Could you check a few things on this drawing? It's one solid part, dimensions in mm from its lowest x, y, z. Give positions to 0.01 mm unless a question says otherwise; leave off trailing zeros. Loops run counter-clockwise (first coordinate to the right, second up) from the corner with the lowest first, then second, coordinate; pieces in that order, holes last. Notation, with made-up numbers: M 50,81.5 L 96,81.5 A21 ccw 96,111.5 Z; hole C 44.25,-7.5 d9. An arc over 180 degrees is marked long. Write each question's results on one line, items separated by ' | '. Start each with the question number.
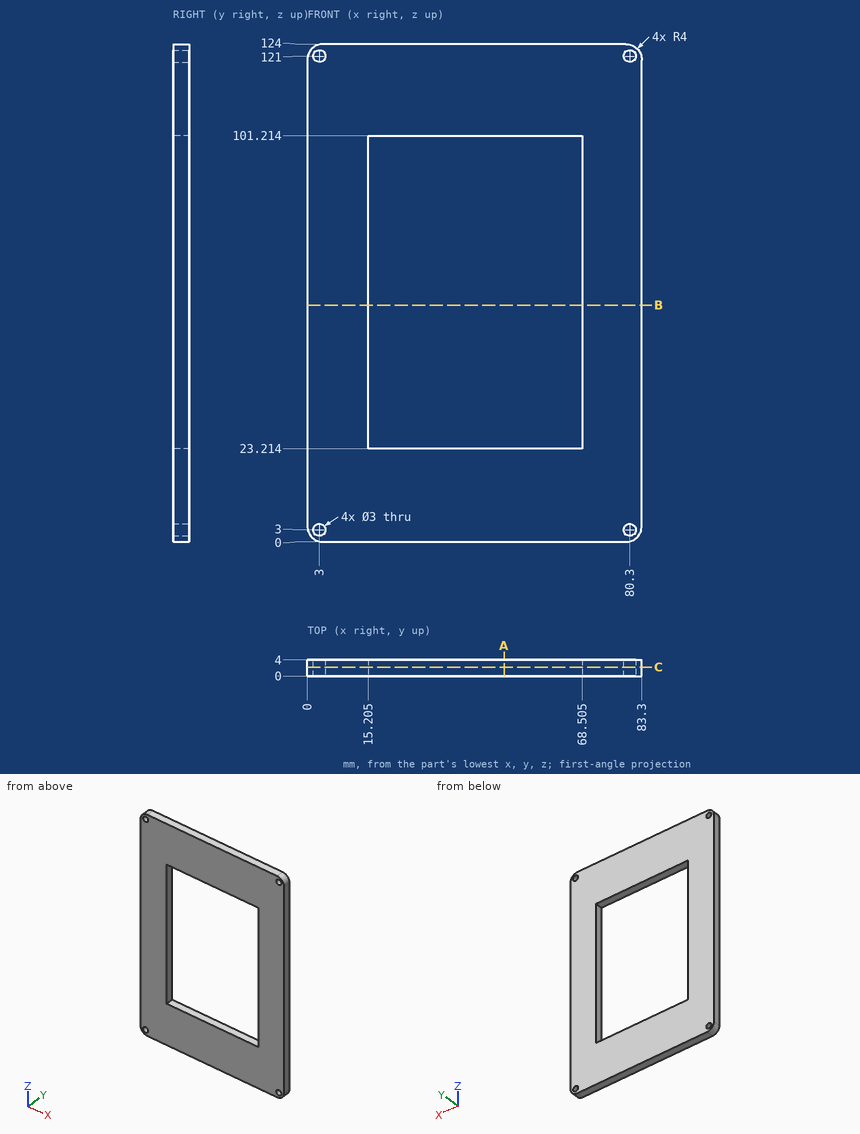
1) If we section it at A-A on x = 49: Write out the boundary of the cut face in (y, z), plus the area to 3 significant figures.
2) I'm going to push a flat-ended pin straight in: P1, Ø1, axis at y = 2, z = 45, coming from the -X side. Where does the tip first touch, or does it pass through?
3) Please list where these lines run through material, in increasing order: line 1 (X direction, y = 3.75, z = 88.5) (3 decimals); line 2 (Z direction, x = 24.5, y = 0.5); line 3 (Z direction, x = 80.3, y = 3.2). Write a range as from..to.
4) If we section it at B-B on z = 59: Write out the boundary of the cut face in (x, y) (3 decimals).
5) If we section it at C-C on y = 2.2: Write out the boundary of the cut face in (x, z) (3 decimals).
Calculated:
1) outline: M 0,0 L 4,0 L 4,23.21 L 0,23.21 Z; M 0,101.21 L 4,101.21 L 4,124 L 0,124 Z | area: 184 mm2
2) P1: stops at x = 0
3) line 1: x = 0..15.205, 68.505..83.3 | line 2: z = 0..23.21, 101.21..124 | line 3: z = 0.13..1.5, 4.5..119.5, 122.5..123.87
4) outline: M 0,0 L 15.205,0 L 15.205,4 L 0,4 Z; M 68.505,0 L 83.3,0 L 83.3,4 L 68.505,4 Z
5) outline: M 0,4 A4 ccw 4,0 L 79.3,0 A4 ccw 83.3,4 L 83.3,120 A4 ccw 79.3,124 L 4,124 A4 ccw 0,120 Z; hole C 3,3 d3; hole C 3,121 d3; hole M 15.205,23.214 L 68.505,23.214 L 68.505,101.214 L 15.205,101.214 Z; hole C 80.3,3 d3; hole C 80.3,121 d3
